For this review, take the finished solid that the model builds, in its own axes (mm). A direction names the side the tool comes from. Round coordinates to 2 decimals unless told otherwise and drop trailing zeros. Order: outer loops, then holes, each group sorted by start corner. A loop starts at its lowest first (then second) coordinate and runs counter-clockwise, first axis right, second up. Notation, with made-up numbers: M 69,22.5 L 118,22.5 A19 ccw 118,26.5 Z; hole C -10,29 d7. An arc over 180 degrees is marked long. Write item = value, one per line. Start each with the question number.
from build123d import *

# Parameters (mm, degrees)
BOSS_EXTRUDE1_DEPTH         = 3
FILLET1_R                   = 10
M3_CLEARANCE_HOLE1_D        = 3.4
CUT_EXTRUDE1_DEPTH          = 61.741531853
SKETCH7_W                   = 13.775
SKETCH7_H                   = 6
SKETCH7_W_2                 = 28.225
BOSS_EXTRUDE2_DEPTH         = 8
SKETCH15_W                  = 10.578557518
SKETCH15_H                  = 3
BOSS_EXTRUDE3_DEPTH         = 10.125
FILLET2_R                   = 2
TAP_DRILL_FOR_M3X0_5_TAP1_D = 2.5


with BuildPart() as part:
    # Sketch1 → Boss-Extrude1 (new body)
    with BuildSketch(Plane.XY):
        Polygon((23.474558014, 7.846809304), (23.474558014, -28.653190696), (53.474558014, -28.653190696), (53.474558014, 12.846809304), (-40.975441986, 12.846809304), (-40.975441986, -28.653190696), (-30.975441986, -28.653190696), (-30.975441986, 7.846809304), align=None)
    extrude(amount=BOSS_EXTRUDE1_DEPTH)

    # Fillet1
    fillet1_edges = [part.edges().sort_by_distance(p)[0] for p in [
        (23.474558014, 7.846809304, 1.5),
        (-30.975441986, 7.846809304, 1.5),
    ]]
    fillet(fillet1_edges, radius=FILLET1_R)

    # M3 Clearance Hole1 (through all)
    with Locations(Plane(origin=(0, 0, 0), x_dir=(-1, 0, 0), z_dir=(0, 0, -1))):
        with Locations((-48.474558014, 7.846809304), (35.975441986, -23.653190696), (35.975441986, 7.846809304), (-48.474558014, -23.653190696), (-29.467521423, -37.965948117)):
            Hole(M3_CLEARANCE_HOLE1_D / 2)

    # Sketch5 → Cut-Extrude1 (cut, through all)
    with BuildSketch(Plane.XY.offset(3)):
        with BuildLine():
            Line((23.474558014, -14.256748214), (23.474558014, -17.232031749))
            ThreePointArc((23.474558014, -17.232031749), (25.270647998, -35.897802119), (42.566674364, -28.653190696))
            Line((42.566674364, -28.653190696), (42.896000496, -28.653190696))
            Line((42.896000496, -28.653190696), (42.896000496, -25.903190696))
            ThreePointArc((42.896000496, -25.903190696), (39.48483647, -17.667912241), (31.249558014, -14.256748214))
            Line((31.249558014, -14.256748214), (23.474558014, -14.256748214))
        make_face()
    extrude(amount=-CUT_EXTRUDE1_DEPTH, mode=Mode.SUBTRACT)

    # Sketch7 → Boss-Extrude2 (add)
    with BuildSketch(Plane.XY.offset(3)):
        with Locations((30.362058014, -5.678190696)):
            Rectangle(SKETCH7_W, SKETCH7_H)
        with Locations((39.362058014, -35.778190696)):
            Rectangle(SKETCH7_W_2, SKETCH7_H)
    extrude(amount=BOSS_EXTRUDE2_DEPTH)


with BuildPart() as boss_extrude2_piece_1:
    # of the separate pieces the step leaves, piece 1, a body of its own (boss_extrude2_pieces)
    add(part.part.solids().sort_by_distance((-20.975441986, 7.846809304, 0))[0])



with BuildPart() as boss_extrude2_piece_2:
    # of the separate pieces the step leaves, piece 2, a body of its own (boss_extrude2_pieces)
    add(part.part.solids().sort_by_distance((53.474558014, -38.778190696, 3))[0])


with BuildPart() as boss_extrude2_piece_1_1:
    add(boss_extrude2_piece_1.part)

    add(boss_extrude2_piece_2.part)  # Boss-Extrude3 merges Boss-Extrude2 piece 2
    # Sketch15 → Boss-Extrude3 (add)
    with BuildSketch(Plane.XZ.offset(28.653190696)):
        with Locations((48.185279255, 1.5)):
            Rectangle(SKETCH15_W, SKETCH15_H)
    extrude(amount=BOSS_EXTRUDE3_DEPTH)

    # Fillet2
    fillet2_edges = [boss_extrude2_piece_1_1.edges().sort_by_distance(p)[0] for p in [
        (53.474558014, -38.778190696, 5.5),
        (48.185279255, -32.778190696, 3),
        (-40.975441986, -28.653190696, 1.5),
        (-40.975441986, 12.846809304, 1.5),
        (53.474558014, 12.846809304, 1.5),
        (-30.975441986, -28.653190696, 1.5),
        (23.474558014, -14.256748214, 1.5),
        (30.362058014, -2.678190696, 3),
        (37.249558014, -5.678190696, 3),
        (30.362058014, -8.678190696, 3),
    ]]
    fillet(fillet2_edges, radius=FILLET2_R)

    # Tap Drill for M3x0.5 Tap1 (through all)
    with Locations(Plane.XY.offset(11)):
        with Locations((31.249558014, -35.778190696), (31.249558014, -5.678190696)):
            Hole(TAP_DRILL_FOR_M3X0_5_TAP1_D / 2)


solid = boss_extrude2_piece_1_1.part
(1) We need section B-B, the plane z = 6.5. Write out the cut boundary in (x, y).
(2) We need section D-D, the plane x = -15. Write out the cut boundary in (y, z), then the cut area to 3 significant figures.
(3) For line 1 along Y through (x, z) = (35, 7.25); line 2 along X through (y, z) = (-36, 8.5); line 3 along Y through (x, z) = (-35, 1.75), list the stretches that pass through material, from the lowest coordinate up.
(4) Draft analysis for pull direction Y (two halves, no side actions). For faces 4 (the cylindrical face through (52.87, 12.28, 1.52)), 5 (the flat face through (30, -8.678, 8)), 6 (the flat face through (-36, -28.653, 1)), state which applies: released by +Y, released by -Y, zero draft, split by the parting line, or undercut.
(5) For faces 1 (the cylindrical face through (39.575, -17.759, 1.521)), 2 (the cylindrical face through (31.47, -9.25, 3.6)), 3 (the flat face through (37.25, -6, 8)), list the 3-axis set-ups (+Z, -Z, +X, -X, +Y, -Y) from which the entire face can be reached by the end or side of a thin tool; tool diameter is ignored.
(6) We need section A-A, the plane y = 3. Write out the cut boundary in (x, z), then the cut area to 3 significant figures.
(7) Insertion check: pin 1 (2.5 mm diameter, centred on x = 0, z = 1.5, fed in from -Y); pin 2 (1.5 mm diameter, centred on x = -36, z = 1.5, fed in from -Y); pin 3 (6 mm diameter, centred on x = 35, z = 7, fed in from +Y). Each pin has a flat end and moves straight along its axis. Give the tip position at first contact, or say it passes through.
(8) We need section C-C, the plane z = 1.75. Write out the cut boundary in (x, y).
Values:
q1.outline = M 23.47,-8.68 L 37.25,-8.68 L 37.25,-2.68 L 23.47,-2.68 Z; M 25.25,-38.78 L 51.47,-38.78 A2 ccw 53.47,-36.78 L 53.47,-32.78 L 25.25,-32.78 Z; hole C 31.25,-35.78 d2.5; hole C 31.25,-5.68 d2.5
q2.outline = M 7.85,0 L 12.85,0 L 12.85,3 L 7.85,3 Z
q2.area = 15.0 mm²
q3.line_1 = -38.78 to -32.78, -8.68 to -2.68
q3.line_2 = 25.25 to 30.02, 32.48 to 53.47
q3.line_3 = -28.65 to -25.05, -22.26 to 6.45, 9.24 to 12.85
q4.face_4 = released by +Y
q4.face_5 = undercut
q4.face_6 = released by -Y
q5.face_1 = +Z, -Z, -Y
q5.face_2 = +Z, +X, -X
q5.face_3 = +Z, +X, +Y
q6.outline = M -40.98,0 L -29.55,0 L -29.55,3 L -40.98,3 Z; M 22.04,0 L 53.47,0 L 53.47,3 L 22.04,3 Z
q6.area = 129 mm²
q7.pin_1 = 7.85
q7.pin_2 = -28.65
q7.pin_3 = -2.41
q8.outline = M -40.98,-26.65 A2 ccw -38.98,-28.65 L -32.98,-28.65 A2 ccw -30.98,-26.65 L -30.98,-2.15 A10 cw -20.98,7.85 L 13.47,7.85 A10 cw 23.47,-2.15 L 23.47,-12.26 A2 ccw 25.47,-14.26 L 31.25,-14.26 A11.65 cw 42.9,-25.9 L 42.9,-38.78 L 51.47,-38.78 A2 ccw 53.47,-36.78 L 53.47,10.85 A2 ccw 51.47,12.85 L -38.98,12.85 A2 ccw -40.98,10.85 Z; hole C -35.98,-23.65 d3.4; hole C -35.98,7.85 d3.4; hole C 31.25,-5.68 d2.5; hole C 48.47,-23.65 d3.4; hole C 48.47,7.85 d3.4
